Build history of the part. All positions in model axes, mm. Round coordinates to 2 decimals unless told otherwise and drop trailing zeros. Loops run counter-clockwise (first coordinate to the right, second up) from the corner with the lowest first, then second, coordinate; pieces in that order, holes last. Notation, with made-up numbers: (87, 46.5) - (118, 46.5) arc R21 cw to (118, 66.5) - close; hole circle Ø1 at (18.5, 14.5). An arc over 180 degrees is marked (long way). Use one line per item in the form item = value. Start each with the question number.
Q1. Saw through at A-A (y = 6.35). Give the cut face in (x, z) (3 decimals), then the cut area to 3 significant figures.
Q2. Saw through at C-C (z = 68.5). Give the cut face in (x, y) (3 decimals), then the cut area to 3 significant figures.
Q3. Pin check, flat tips, straight feed: pin 1 (6 mm diameter, centred on x = -7, z = 40, fed in from +Y); pin 2 (5 mm diameter, centred on x = -60.5, z = 33, fed in from +Y); pin 3 (6 mm diameter, centred on x = -6, y = 8, fed in from +Z); pin 4 (3 mm diameter, centred on x = -21, z = 90.5, fed in from -Y). Stop position of each tip, or through.
Q4. Saw through at B-B (z = 107.95). Give the cut face in (x, y) (3 decimals).
Q5. Drill centre lines: line 1 (Y direction, x = 1, z = 19); line 2 (Y direction, x = 1.75, z = 19.05); line 3 (X direction, y = 4.5, z = 79.5) (3 decimals). Where is each one in solid material? Low to high.
Q6. Saw through at D-D (y = 15.5). Give the cut face in (x, z), then the cut area to 3 significant figures.
Q7. Mould opens along Y. For faces 1 (the face through (1.565, 6.471, 105.203)), 2 (the face through (-72.147, 24.347, 62.611)), 3 (the face through (0, 5, 63)) say: released by +Y, released by -Y, zero draft, split by the parting line, or undercut.
```python
from build123d import *

# Parameters (mm, degrees)
BOSS_EXTRUDE1_DEPTH  = 127
M5_CLEARANCE_HOLE1_D = 5.5


with BuildPart() as part:
    # Sketch1 → Boss-Extrude1 (new body)
    with BuildSketch(Plane.XY):
        Polygon((0, 0), (0, 10.035858671), (-72.418683744, 22.805226522), (-71.86735078, 25.931991138), (3.175, 12.7), (3.175, 0), align=None)
    extrude(amount=BOSS_EXTRUDE1_DEPTH)

    # M5 Clearance Hole1 (through all)
    with Locations(Plane(origin=(3.175, 0, 0), x_dir=(0, 0, -1), z_dir=(1, 0, 0))):
        with Locations((-107.95, 6.35), (-19.05, 6.35)):
            Hole(M5_CLEARANCE_HOLE1_D / 2)


solid = part.part
```
Report:
q1.outline = (0, 0) - (3.175, 0) - (3.175, 16.3) - (0, 16.3) - close; (0, 21.8) - (3.175, 21.8) - (3.175, 105.2) - (0, 105.2) - close; (0, 110.7) - (3.175, 110.7) - (3.175, 127) - (0, 127) - close
q1.area = 368 mm²
q2.outline = (-72.419, 22.805) - (0, 10.036) - (0, 0) - (3.175, 0) - (3.175, 12.7) - (-71.867, 25.932) - close
q2.area = 274 mm²
q3.pin_1 = 15.02
q3.pin_2 = 24.37
q3.pin_3 = through
q3.pin_4 = 13.47
q4.outline = (-72.419, 22.805) - (0, 10.036) - (0, 9.1) - (3.175, 9.1) - (3.175, 12.7) - (-71.867, 25.932) - close; (0, 0) - (3.175, 0) - (3.175, 3.6) - (0, 3.6) - close
q5.line_1 = 0 to 3.6, 9.1 to 13.08
q5.line_2 = 0 to 3.6, 9.1 to 12.95
q5.line_3 = 0 to 3.175
q6.outline = (-30.99, 0) - (-12.7, 0) - (-12.7, 127) - (-30.99, 127) - close
q6.area = 2,320 mm²
q7.face_1 = undercut
q7.face_2 = released by +Y
q7.face_3 = zero draft
